Input: part model. Units: mm. Frame: model coordinates. A direction names the side the tool comes from. Give positions to 0.01 mm unless a question says otherwise; leave off trailing zeros. Loops run counter-clockwise (first coordinate to the right, second up) from the corner with the lowest first, then second, coordinate; pieces in that order, holes last. Notation, with made-up numbers: (5, -38.75) - (63, -38.75) arc R17 cw to (63, -21.75) - close; hole circle Ø1 at (-27.75, 19.25). An arc over 180 degrees is marked (long way). Answer as a JSON object with one key per item and string values. Group by question number.
(1) Section query B-B (z = 31). Return loops of the section in (x, y).
(2) Pin query (flat end, axial travel): P1, Ø1.1, axis at x = -30.5, y = -1.5, coming from the +Z side (3 decimals); P2, Ø3, axis at x = -31, y = -2.5, coming from the -Z side (3 decimals); P3, Ø1, axis at x = -15.5, z = 13, coming from the +Y side; P4, Ø1.5, axis at y = -1.5, z = -44, coming from the -X side. Return the tip coordinate at first contact, or that it passes through.
(3) Mould query, pull axis X, two halves, no side actions, for faces 5 (the flat face through (19.406, -3, 1)), 6 (the flat face through (-13.614, -3, 0)), 7 (the flat face through (21, -3, 67.31)), 8 (the flat face through (-19, -3, 9.271)). Classes: +X half, -X half, draft (parallel to the pull), parting line (faces both ways), or undercut.
(4) Material intervals for L1, parallel to Z at x = -30, y = -2 (3 decimals); L2, parallel to X at y = -2.1, z = 7; L3, parallel to X at y = -3.65, z = -63.5, sorted ascending.
(5) Access query for faces 1 (the flat face through (21, -3, -67.31)), 2 (the flat face through (-24.79, -3, -13)), 3 (the flat face through (-31, -3, -57.785)), 4 (the flat face through (-32.664, -3, -34)). Directions: +Z, -Z, +X, -X, +Y, -Y. A direction counts if a zero-diameter tool reaches every point of the face in a straight line with its end or side. Return the directions, or none.
(6) Section query A-A (x = -23). Return loops of the section in (y, z), plus the area to 3 significant figures.
```python
from build123d import *

# Parameters (mm, degrees)
F0_W     = 3.81
F0_H     = 10.16
F2_DEPTH = 5.08
F1_W     = 3.0988
F1_H     = 67.31
F1_W_2   = 4.064
F1_H_2   = 7.62
F1_W_3   = 2.032
F1_H_3   = 9.271
F3_DEPTH = 33.274


with BuildPart() as f2:
    # F0 (on Front) → F2 (new body)
    with BuildSketch(Plane.XZ):
        Polygon((28.8544, 71.12), (-28.8544, 71.12), (-28.8544, 57.785), (-28.8544, 47.625), (-28.8544, 38.6334), (-28.8544, 28.4734), (-28.8544, 0), (-28.8544, -28.4734), (-28.8544, -38.6334), (-28.8544, -47.625), (-28.8544, -57.785), (-28.8544, -71.12), (28.8544, -71.12), align=None)
        with Locations((-30.7594, 52.705)):
            Rectangle(F0_W, F0_H)
        with Locations((-30.7594, 33.5534)):
            Rectangle(F0_W, F0_H)
        with Locations((-30.7594, -52.705)):
            Rectangle(F0_W, F0_H)
        with Locations((-30.7594, -33.5534)):
            Rectangle(F0_W, F0_H)
    extrude(amount=F2_DEPTH)

    # F1 (on Front) → F3 (cut)
    with BuildSketch(Plane.XZ):
        with Locations((20.955, 33.655)):
            Rectangle(F1_W, F1_H)
        with Locations((20.955, -33.655)):
            Rectangle(F1_W, F1_H)
        Polygon((-13.6144, -9.271), (-13.6144, 0), (-13.6144, 9.271), (-24.7904, 9.271), (-26.8224, 9.271), (-26.8224, 0), (-28.8544, 0), (-28.8544, -9.271), (-24.7904, -9.271), align=None)
        Polygon((-26.8224, 9.271), (-24.7904, 9.271), (-24.7904, 16.891), (-28.8544, 16.891), (-28.8544, 9.271), align=None)
        with Locations((-26.8224, -13.081)):
            Rectangle(F1_W_2, F1_H_2)
        with Locations((-27.8384, 4.6355)):
            Rectangle(F1_W_3, F1_H_3)
    extrude(amount=F3_DEPTH, mode=Mode.SUBTRACT)


solid = f2.part
```
Recorded:
{
 "1": {"outline": "(-32.66, -5.08) - (19.41, -5.08) - (19.41, 0) - (-32.66, 0) - close; (22.5, -5.08) - (28.85, -5.08) - (28.85, 0) - (22.5, 0) - close"},
 "2": {"P1": "stops at z = 57.785", "P2": "stops at z = -57.785", "P3": "stops at y = 0", "P4": "stops at x = -28.85"},
 "3": {"face 5": "undercut", "face 6": "-X half", "face 7": "undercut", "face 8": "draft"},
 "4": {"L1": "z = -57.785 to -47.625, -38.633 to -28.473, 28.473 to 38.633, 47.625 to 57.785", "L2": "x = -13.61 to 19.41, 22.5 to 28.85", "L3": "x = -28.85 to 19.41, 22.5 to 28.85"},
 "5": {"face 1": "+Y, -Y", "face 2": "-X, +Y, -Y", "face 3": "-Z, -X, +Y, -Y", "face 4": "+Z, -Z, -X, +Y, -Y"},
 "6": {"outline": "(-5.08, -71.12) - (0, -71.12) - (0, -9.27) - (-5.08, -9.27) - close; (-5.08, 9.27) - (0, 9.27) - (0, 71.12) - (-5.08, 71.12) - close", "area": "628 mm^2"}
}
